from build123d import *

# Parameters (mm, degrees)
SKETCH038_R   = 10
SKETCH038_R_2 = 6
PAD014_DEPTH  = 2


with BuildPart() as bearing_inner_back_left:
    # Sketch038 → Pad014 (new body)
    with BuildSketch(Plane.YZ):
        Circle(SKETCH038_R)
        Circle(SKETCH038_R_2, mode=Mode.SUBTRACT)
    extrude(amount=PAD014_DEPTH)


with BuildPart() as bearing_inner_back_left_1:
    # Body010 placement: moved
    add(bearing_inner_back_left.part.moved(Location((10, 51, -44))))


with BuildPart() as bearing_inner_front_left:
    # Part__Mirroring010: instance of bearing-inner-back-left
    add(bearing_inner_back_left_1.part.mirror(Plane(origin=(11, -4e-06, -44.000004), x_dir=(1, 0, 0), z_dir=(0, 1, 0))))


with BuildPart() as bearing_inner_front_right:
    # Part__Mirroring011: instance of bearing-inner-front-left
    add(bearing_inner_front_left.part.mirror(Plane(origin=(0, 0, 0), x_dir=(0, -1, 0), z_dir=(1, 0, 0))))


solid = bearing_inner_front_right.part
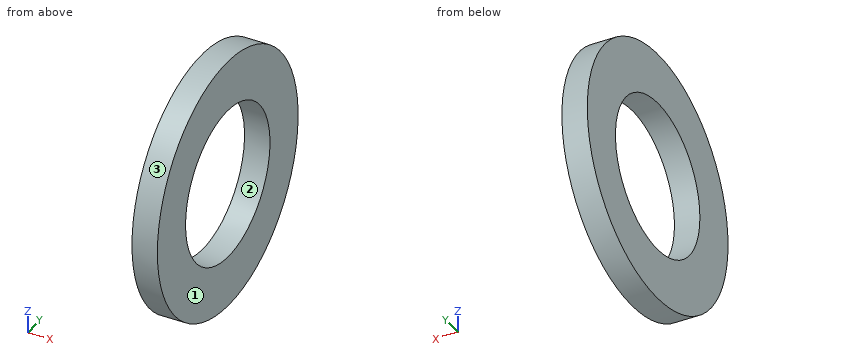
Verification items for the finished model (mm, model axes). Face numbers are marked on the shaded views. Coordinates: 2 decimals unless noted, no trailing zeros. Order: outer loops, then holes, each group sorted by start corner. A loop starts at its lowest first (then second) coordinate and runs counter-clockwise, first axis right, second up. Notation, with made-up numbers: M 74.25,47.5 L 115.25,47.5 A14 cw 115.25,69.5 Z; hole C -26.75,60 d11. An arc over 180 degrees is marked long. One line per item, written item: value. Start each with the question number.
Item 1: Sectioned sample at D-D on z = -51.5. Record the cut outline in (x, y), then the cut area to 3 significant figures.
Item 2: Sectioned sample at C-C on y = -48. Record the cut outline in (x, z), then the cut area to 3 significant figures.
Item 3: Sectioned sample at A-A on z = -44. Record the cut outline in (x, y).
Item 4: Mould release check, pull along Z, two halves, no side actions. Record for the marked faces 1, 2 and 3: pulls with the +Z half, pulls with the -Z half, needs draft (parallel to the pull), parting line crosses it, or undercut.
Item 5: Thickness scan on probe 1 along Z at (x, y) = (-11.8, -51); probe 2 along Z at (x, y) = (-10.4, -47.25); probe 3 along Y at (x, z) = (-10.15, -40.5). Record the ranges inside material, lowest first.
Item 6: Sectioned sample at B-B on x = -11.15. Record the cut outline in (y, z), then the cut area to 3 significant figures.
Calculated:
1. outline: M -12,-57.61 L -10,-57.61 L -10,-44.39 L -12,-44.39 Z
1. area: 26.5 mm^2
2. outline: M -12,-53.54 L -10,-53.54 L -10,-49.2 L -12,-49.2 Z; M -12,-38.8 L -10,-38.8 L -10,-34.46 L -12,-34.46 Z
2. area: 17.4 mm^2
3. outline: M -12,-61 L -10,-61 L -10,-57 L -12,-57 Z; M -12,-45 L -10,-45 L -10,-41 L -12,-41 Z
4. face 1: needs draft
4. face 2: undercut
4. face 3: parting line crosses it
5. probe 1: -54 to -50, -38 to -34
5. probe 2: -53.27 to -48.68, -39.32 to -34.73
5. probe 3: -60.37 to -55.87, -46.13 to -41.63
6. outline: C -51,-44 d20; hole C -51,-44 d12
6. area: 201 mm^2
